Work out the finished part from the listing and answer in its coordinate system (mm). Round coordinates to 2 decimals unless told otherwise and drop trailing zeros. Order: outer loops, then holes, each group sorted by start corner. A loop starts at its lowest first (then second) coordinate and runs counter-clockwise, first axis right, second up. Notation, with made-up numbers: (-9, 23) - (7, 23) arc R20 ccw to (7, 40) - close; hole circle Ø2 at (88.5, 32). An arc over 180 degrees is marked (long way). Answer in a Markdown table with one row per item.
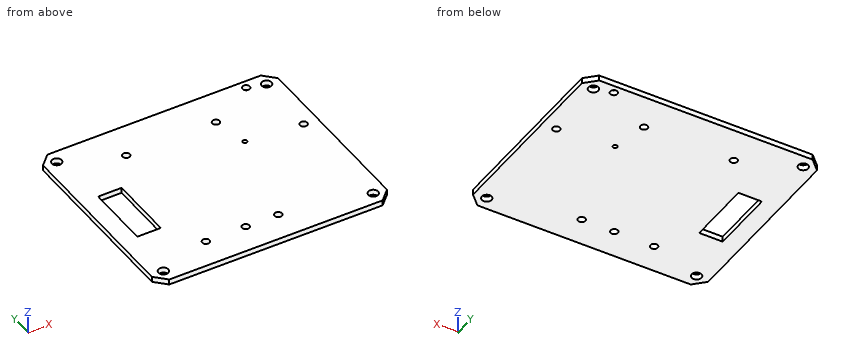
Autodesk Inventor part; units mm, degrees
ref_plane "YZ Plane" through (0, 0, 0) normal (1, 0, 0) x (0, 1, 0)
ref_plane "XZ Plane" through (0, 0, 0) normal (0, 1, 0) x (-1, 0, 0)
ref_plane "XY Plane" through (0, 0, 0) normal (0, 0, 1) x (1, 0, 0)
sketch "Эскиз1" plane through (0, 0, 0) normal (0, 0, 1) x (1, 0, 0)
  line L0 (-73.63, -2.23) -> (5.37, -2.23)
  arc A0 (5.37, -2.23) -> (8.37, 0.77) centre (5.37, 0.77) ccw
  line L1 (8.37, 0.77) -> (8.37, 50.77)
  arc A1 (8.37, 50.77) -> (5.37, 53.77) centre (5.37, 50.77) ccw
  line L2 (5.37, 53.77) -> (-73.63, 53.77)
  arc A2 (-73.63, 53.77) -> (-76.63, 50.77) centre (-73.63, 50.77) ccw
  line L3 (-76.63, 50.77) -> (-76.63, 0.77)
  arc A3 (-76.63, 0.77) -> (-73.63, -2.23) centre (-73.63, 0.77) ccw
  circle A4 centre (4.87, 50.27) radius 1.35
  circle A5 centre (-53.13, 50.27) radius 1.35
  circle A6 centre (0.07, 48.67) radius 0.325
  circle A7 centre (-5.73, 48.67) radius 0.325
  circle A8 centre (-68.88, 49.235) radius 1.65
  circle A9 centre (4.87, 44.27) radius 1.55
  circle A10 centre (-68.88, 37.805) radius 1.65
  circle A11 centre (-53.13, 7.27) radius 1.55
  circle A12 centre (4.87, 1.27) radius 1.35
  circle A13 centre (-53.13, 1.27) radius 1.35
  line L4 (5.37, -2.23) -> (8.37, -2.23) construction
  line L5 (8.37, -2.23) -> (8.37, 0.77) construction
  line L6 (8.37, 0.77) -> (5.37, 0.77) construction
  line L7 (5.37, 0.77) -> (5.37, -2.23) construction
  line L8 (8.37, -2.23) -> (-56.63, -2.23)
  line L9 (-56.63, -2.23) -> (-56.63, 53.77)
  line L10 (-56.63, 53.77) -> (8.37, 53.77)
  line L11 (8.37, 53.77) -> (8.37, -2.23)
  line L12 (8.37, -2.23) -> (-56.63, -2.23)
  line L13 (-56.63, -2.23) -> (-56.63, -13.23)
  line L14 (-56.63, -13.23) -> (8.37, -13.23)
  line L15 (8.37, -13.23) -> (8.37, -2.23)
  line L16 (-56.63, 53.77) -> (8.37, 53.77)
  line L17 (8.37, 53.77) -> (8.37, 61.77)
  line L18 (8.37, 61.77) -> (-56.63, 61.77)
  line L19 (-56.63, 61.77) -> (-56.63, 53.77)
  line L20 (0.1, 51.34) -> (-0.1, 51.34) construction
  line L21 (-0.1, 51.34) -> (-0.1, 51.74) construction
  line L22 (0.1, 51.74) -> (-0.1, 51.74) construction
  line L23 (0.1, 51.34) -> (0.1, 51.74) construction
  line L24 (0, 51.74) -> (0, 51.34) construction
  line L25 (0.1, 51.54) -> (-0.1, 51.54) construction
  circle A14 centre (0, 51.54) radius 1
  line L26 (4.5478, 32.4872) -> (4.3622, 32.4872) construction
  line L27 (4.3622, 32.4872) -> (4.3622, 32.6728) construction
  line L28 (4.3622, 32.6728) -> (4.5478, 32.6728) construction
  line L29 (4.5478, 32.6728) -> (4.5478, 32.4872) construction
  line L30 (4.455, 32.4872) -> (4.455, 32.6728) construction
  line L31 (4.5478, 32.58) -> (4.3622, 32.58) construction
  circle A15 centre (4.455, 32.58) radius 1
  line L32 (-37.8578, 43.7922) -> (-37.8578, 43.9778) construction
  line L33 (-37.8578, 43.9778) -> (-37.6722, 43.9778) construction
  line L34 (-37.6722, 43.9778) -> (-37.6722, 43.7922) construction
  line L35 (-37.6722, 43.7922) -> (-37.8578, 43.7922) construction
  line L36 (-37.765, 43.7922) -> (-37.765, 43.9778) construction
  line L37 (-37.6722, 43.885) -> (-37.8578, 43.885) construction
  circle A16 centre (-37.765, 43.885) radius 1
  line L38 (-14.8578, 43.7922) -> (-14.8578, 43.9778) construction
  line L39 (-14.8578, 43.9778) -> (-14.6722, 43.9778) construction
  line L40 (-14.6722, 43.9778) -> (-14.6722, 43.7922) construction
  line L41 (-14.6722, 43.7922) -> (-14.8578, 43.7922) construction
  line L42 (-14.765, 43.7922) -> (-14.765, 43.9778) construction
  line L43 (-14.6722, 43.885) -> (-14.8578, 43.885) construction
  circle A17 centre (-14.765, 43.885) radius 1 construction
  circle A18 centre (-10.9214, 33.9778) radius 0.85 construction
  circle A19 centre (-10.9214, 33.9778) radius 0.6
  line L44 (-18.88, 5.47) -> (-18.38, 5.47) construction
  line L45 (-18.88, 5.47) -> (-18.88, 6.22) construction
  line L46 (-18.88, 6.22) -> (-18.38, 6.22) construction
  line L47 (-18.38, 5.47) -> (-18.38, 6.22) construction
  line L48 (-27.88, 5.47) -> (-27.38, 5.47) construction
  line L49 (-27.88, 5.47) -> (-27.88, 6.22) construction
  line L50 (-27.88, 6.22) -> (-27.38, 6.22) construction
  line L51 (-27.38, 5.47) -> (-27.38, 6.22) construction
  line L52 (-38.88, 5.47) -> (-38.38, 5.47) construction
  line L53 (-38.88, 5.47) -> (-38.88, 6.22) construction
  line L54 (-38.88, 6.22) -> (-38.38, 6.22) construction
  line L55 (-38.38, 5.47) -> (-38.38, 6.22) construction
  line L56 (-18.38, 5.845) -> (-18.88, 5.845) construction
  line L57 (-18.63, 5.47) -> (-18.63, 6.22) construction
  circle A20 centre (-18.63, 5.845) radius 1
  line L58 (-27.38, 5.845) -> (-27.88, 5.845) construction
  line L59 (-27.63, 5.47) -> (-27.63, 6.22) construction
  line L60 (-38.38, 5.845) -> (-38.88, 5.845) construction
  line L61 (-38.63, 5.47) -> (-38.63, 6.22) construction
  circle A21 centre (-38.63, 5.845) radius 1
  circle A22 centre (-27.63, 5.845) radius 1
  line L62 (-14.765, 43.885) -> (-12.965, 43.885) construction
  circle A23 centre (-12.965, 43.885) radius 1
  line L63 (-56.63, 53.77) -> (-51.63, 53.77) construction
  line L64 (-51.63, 53.77) -> (-51.63, 33.773) construction
  line L65 (-51.63, 33.773) -> (-56.63, 33.773) construction
  line L66 (-56.63, 33.773) -> (-56.63, 53.77) construction
  line L67 (-51.63, 33.773) -> (-45.13, 33.773)
  line L68 (-45.13, 33.773) -> (-45.13, 15.773)
  line L69 (-45.13, 15.773) -> (-51.63, 15.773)
  line L70 (-51.63, 15.773) -> (-51.63, 33.773)
  point P0 (0, 0)
  point P1 (8.37, 0.77)
  point P2 (8.37, 53.77)
  dimension "d0" = 65
  dimension "d1" = 56
  dimension "d8" = 65
  dimension "d9" = 11
  dimension "d10" = 8
  dimension "d11" = 2
  dimension "d12" = 2
  dimension "d13" = 2
  dimension "d14" = 2
  dimension "d15" = 2
  dimension "d16" = 2
  dimension "d17" = 2
  dimension "d21" = 1.8
  dimension "d22" = 2
  dimension "d23" = 5
  dimension "d24" = 19.997
  dimension "d25" = 6.5
  dimension "d26" = 18
extrude "Выдавливание1" add sketch "Эскиз1" along normal blind 1.5 contours L9 L2 A1 L1 A0 L0 | A0 L11 L8 | L10 L11 A1 | A6 | A7 | A9 | A11
chamfer "Фаска1" distance 3 angle 45 4 edges at (8.37, -2.23, 0.75) (8.37, 53.77, 0.75) (-56.63, 53.77, 0.75) (-56.63, -2.23, 0.75)
properties part number "board_rpi"
1) Find section B-B, the plane z = 0.95. Give the number of separate pieces and of enclosed holes in the cut face, then the cut area to 3 significant figures.
Filled in:
| item | result |
|---|---|
| separate pieces | 1 |
| enclosed holes | 13 |
| area | 3,460 mm^2 |
2) Find the intervals of material crossed by probe 1 along X at (y, z) = (6, 1.15); probe 2 along Y at (x, z) = (-53, 1.4); probe 3 along Y at (x, z) = (-13, 1.15), in increasing order. Write a range as from..to.
Filled in:
| item | result |
|---|---|
| probe 1 | x = -56.63..-39.62, -37.64..-28.62, -26.64..-19.62, -17.64..8.37 |
| probe 2 | y = -2.23..-0.07, 2.61..48.93, 51.61..53.77 |
| probe 3 | y = -2.23..42.89, 44.88..53.77 |
3) Find section A-A, the plane x = -18.63. Give the vertices of the cut face in (y, z) (3 decimals).
Filled in:
| item | result |
|---|---|
| outline | (-2.23, 0) - (4.845, 0) - (4.845, 1.5) - (-2.23, 1.5) - close; (6.845, 0) - (53.77, 0) - (53.77, 1.5) - (6.845, 1.5) - close |
